from build123d import *

# Parameters (mm, degrees)
SKETCH_W        = 180
SKETCH_H        = 74
PAD_DEPTH       = 30
SKETCH001_W     = 170
SKETCH001_H     = 23
POCKET_DEPTH    = 71
SKETCH002_W     = 40
SKETCH002_H     = 12.5
POCKET001_DEPTH = 5
SKETCH003_W     = 40
SKETCH003_H     = 8
POCKET002_DEPTH = 200
SKETCH004_W     = 150
SKETCH004_H     = 62
POCKET003_DEPTH = 5
SKETCH005_W     = 100
SKETCH005_H     = 10
POCKET004_DEPTH = 1.7
SKETCH006_R     = 6
POCKET005_DEPTH = 5
FILLET_R        = 2.5
FILLET001_R     = 1.5
FILLET002_R     = 2.5
FILLET003_R     = 1.5


with BuildPart() as part:
    # Sketch → Pad (new body)
    with BuildSketch(Plane.XY):
        Rectangle(SKETCH_W, SKETCH_H)
    extrude(amount=PAD_DEPTH)

    # Sketch001 (on Face3 of Pad) → Pocket (cut)
    with BuildSketch(Plane(origin=(0, 37, 0), x_dir=(-1, 0, 0), z_dir=(0, 1, 0))):
        with Locations((0, 15)):
            Rectangle(SKETCH001_W, SKETCH001_H)
    extrude(amount=-POCKET_DEPTH, mode=Mode.SUBTRACT)

    # Sketch002 (on Face3 of Pocket) → Pocket001 (cut)
    with BuildSketch(Plane.YZ.offset(90)):
        with Locations((0, 9.75)):
            Rectangle(SKETCH002_W, SKETCH002_H)
    extrude(amount=-POCKET001_DEPTH, mode=Mode.SUBTRACT)

    # Sketch003 (on Face2 of Pocket001) → Pocket002 (cut)
    with BuildSketch(Plane(origin=(-90, 0, 0), x_dir=(0, -1, 0), z_dir=(-1, 0, 0))):
        with Locations((0, 20)):
            Rectangle(SKETCH003_W, SKETCH003_H)
    extrude(amount=-POCKET002_DEPTH, mode=Mode.SUBTRACT)

    # Sketch004 (on Face5 of Pocket002) → Pocket003 (cut)
    with BuildSketch(Plane.XY.offset(30)):
        Rectangle(SKETCH004_W, SKETCH004_H)
    extrude(amount=-POCKET003_DEPTH, mode=Mode.SUBTRACT)

    # Sketch005 (on Face4 of Pocket003) → Pocket004 (cut)
    with BuildSketch(Plane(origin=(0, 0, 0), x_dir=(1, 0, 0), z_dir=(0, 0, -1))):
        with Locations((-30, 22)):
            Rectangle(SKETCH005_W, SKETCH005_H)
    extrude(amount=-POCKET004_DEPTH, mode=Mode.SUBTRACT)

    # Sketch006 → Pocket005 (cut)
    with BuildSketch(Plane.XY.offset(3.5)):
        with Locations((21.5, -4.5)):
            Circle(SKETCH006_R)
    extrude(amount=-POCKET005_DEPTH, mode=Mode.SUBTRACT)

    # Fillet
    fillet_edges = [part.edges().sort_by_distance(p)[0] for p in [
        (90, 37, 15),
        (90, -37, 15),
        (-90, 37, 15),
        (-90, -37, 15),
    ]]
    fillet(fillet_edges, radius=FILLET_R)

    # Fillet001
    fillet001_edges = [part.edges().sort_by_distance(p)[0] for p in [
        (87.5, 20, 24),
        (87.5, -20, 24),
        (87.5, -20, 3.5),
        (87.5, 20, 3.5),
        (90, 0, 24),
        (90, 20, 13.75),
        (90, 0, 3.5),
        (90, -20, 13.75),
        (-90, 20, 20),
        (-90, 0, 16),
        (-90, 0, 24),
        (-90, -20, 20),
        (-87.5, 20, 24),
        (-87.5, -20, 24),
        (-87.5, -20, 16),
        (-87.5, 20, 16),
    ]]
    fillet(fillet001_edges, radius=FILLET001_R)

    # Fillet002
    fillet002_edges = [part.edges().sort_by_distance(p)[0] for p in [
        (-75, 31, 28.25),
        (-75, -31, 28.25),
        (75, 31, 28.25),
        (75, -31, 28.25),
    ]]
    fillet(fillet002_edges, radius=FILLET002_R)

    # Fillet003
    fillet003_edges = [part.edges().sort_by_distance(p)[0] for p in [
        (-75, 0, 30),
        (0, 31, 30),
        (75, 0, 30),
        (0, -31, 30),
    ]]
    fillet(fillet003_edges, radius=FILLET003_R)


solid = part.part
Check sheet for the modelled part. Datum: model origin and axes. Units: mm. A direction names the side the tool comes from. Give positions to 0.01 mm unless a question says otherwise; leave off trailing zeros. Loops run counter-clockwise (first coordinate to the right, second up) from the corner with the lowest first, then second, coordinate; pieces in that order, holes last. Notation, with made-up numbers: M 48.5,87.5 L 76.5,87.5 A13 ccw 76.5,93.5 Z; hole C -2,25.5 d1. An arc over 180 degrees is marked long. Use a Markdown table: item, result. Add a question column.
Q1. Go/stop test with flat-tipped pins: pin 1 (1 mm diameter, centred on x = -86.5, y = -2.5, fed in from -Z); pin 2 (5 mm diameter, centred on y = 6.5, z = 10.5, fed in from +X); pin 3 (21.5 mm diameter, centred on x = -1, y = -1.5, fed in from +Z). Record where each tip stops, or that it passes through.
Q2. Sectioned sample at C-C, the plane y = -4.5. Record the cut outline in (x, z), then the cut area to 3 significant figures.
Q3. Mould release check, pull along Z, two halves, no side actions. Record for faces 5 (the flat face through (0, 33, 26.5)), 6 (the flat face through (0, 33, 30)), 7 (the flat face through (87, 20, 14)), 8 (the flat face through (-90, 0, 11)): pulls with the +Z half, pulls with the -Z half, needs draft (parallel to the pull), parting line crosses it, or undercut.
Q4. Sectioned sample at D-D, the plane x = 42. Record the cut outline in (y, z), then the cut area to 3 significant figures.
Q5. Tool access check on faces 1 (the flat face through (-87, 20, 20)), 2 (the flat face through (1, -34, 15)), 3 (the flat face through (87, -20, 14)), 4 (the cylindrical face through (16.74, -8.15, 1.77)). Record the directions out of +Z, -Z, +X, -X, +Y, -Y that give a thin tool (end or side, any length) a straight path to the whole face; none if there is none.
Q6. Sectioned sample at A-A, the plane x = -26. Record the cut outline in (y, z), then the cut area to 3 significant figures.
Q7. Scan lines: line 1 along Y through (x, z) = (21.5, 2.75); line 2 along Z through (x, y) = (-36, 34); line 3 along Y through (x, z) = (-56, 28). Record each from-to range of solid material in increasing order. Write a range as [from, to].
Q8. Sectioned sample at B-B, the plane y = 6. Record the cut outline in (x, z), then the cut area to 3 significant figures.
Verdict:
| question | item | result |
|---|---|---|
| 1 | pin 1 | z = 0 |
| 1 | pin 2 | x = -85 |
| 1 | pin 3 | z = 3.5 |
| 2 | outline | M -90,0 L 15.5,0 L 15.5,3.5 L -85,3.5 L -85,16 L -88.5,16 A1.5 ccw -90,14.5 Z; M -90,25.5 A1.5 ccw -88.5,24 L -85,24 L -85,26.5 L -75,26.5 L -75,28.5 A1.5 ccw -76.5,30 L -90,30 Z; M 27.5,0 L 90,0 L 90,2 A1.5 ccw 88.5,3.5 L 27.5,3.5 Z; M 75,26.5 L 85,26.5 L 85,24 L 88.5,24 A1.5 ccw 90,25.5 L 90,30 L 76.5,30 A1.5 ccw 75,28.5 Z |
| 2 | area | 778 mm^2 |
| 3 | face 5 | undercut |
| 3 | face 6 | pulls with the +Z half |
| 3 | face 7 | undercut |
| 3 | face 8 | needs draft |
| 4 | outline | M -37,0 L 37,0 L 37,3.5 L -34,3.5 L -34,26.5 L -31,26.5 L -31,28.5 A1.5 ccw -32.5,30 L -37,30 Z; M 31,26.5 L 37,26.5 L 37,30 L 32.5,30 A1.5 ccw 31,28.5 Z |
| 4 | area | 369 mm^2 |
| 5 | face 1 | +X, -X |
| 5 | face 2 | +Y |
| 5 | face 3 | +X |
| 5 | face 4 | +Z, -Z |
| 6 | outline | M -37,0 L -27,0 L -27,1.7 L -17,1.7 L -17,0 L 37,0 L 37,3.5 L -34,3.5 L -34,26.5 L -31,26.5 L -31,28.5 A1.5 ccw -32.5,30 L -37,30 Z; M 31,26.5 L 37,26.5 L 37,30 L 32.5,30 A1.5 ccw 31,28.5 Z |
| 6 | area | 352 mm^2 |
| 7 | line 1 | [-37, -10.5], [1.5, 37] |
| 7 | line 2 | [0, 3.5], [26.5, 30] |
| 7 | line 3 | [-37, -31], [31, 37] |
| 8 | outline | M -90,0 L 90,0 L 90,2 A1.5 ccw 88.5,3.5 L -85,3.5 L -85,16 L -88.5,16 A1.5 ccw -90,14.5 Z; M -90,25.5 A1.5 ccw -88.5,24 L -85,24 L -85,26.5 L -75,26.5 L -75,28.5 A1.5 ccw -76.5,30 L -90,30 Z; M 75,26.5 L 85,26.5 L 85,24 L 88.5,24 A1.5 ccw 90,25.5 L 90,30 L 76.5,30 A1.5 ccw 75,28.5 Z |
| 8 | area | 820 mm^2 |
